Here's how the part is built. I have some questions about the finished solid (model axes, mm). A direction names the side the tool comes from. Give positions to 0.01 mm unless a question says otherwise; leave off trailing zeros. Loops run counter-clockwise (first coordinate to the right, second up) from the corner with the lowest first, then second, coordinate; pieces in that order, holes last. Notation, with made-up numbers: (5, 46.25) - (35, 46.25) arc R19 cw to (35, 65.25) - close; hole circle Ø4 at (50, 72.5). An arc over 180 degrees is marked (long way). Use a Markdown table: item, result.
from build123d import *

# Parameters (mm, degrees)
SKETCH2_W             = 40.64
SKETCH2_H             = 26.67
BOSS_EXTRUDE1_DEPTH   = 37.338
SKETCH3_R             = 3.7592
BODY_TUBE_CUT_DEPTH   = 62.294573528
SKETCH4_W             = 22.86
SKETCH4_H             = 18.288
SERVO_BODY_HOLE_DEPTH = 26.67
CUT_EXTRUDE3_REACH    = 63.295
SKETCH5_W             = 7.874
SKETCH5_H             = 9.144


with BuildPart() as part:
    # Sketch2 → Boss-Extrude1 (new body)
    with BuildSketch(Plane(origin=(0, 0, 0), x_dir=(1, 0, 0), z_dir=(0, 1, 0))):
        with Locations((20.32, 13.335)):
            Rectangle(SKETCH2_W, SKETCH2_H)
    extrude(amount=BOSS_EXTRUDE1_DEPTH)

    # Sketch3 → Body Tube Cut (cut, through all)
    with BuildSketch(Plane(origin=(40.64, 0, 0), x_dir=(0, 0, -1), z_dir=(1, 0, 0))):
        with Locations((13.335, 0)):
            Circle(SKETCH3_R)
    extrude(amount=-BODY_TUBE_CUT_DEPTH, mode=Mode.SUBTRACT)

    # Sketch4 → Servo Body Hole (cut)
    with BuildSketch(Plane.XY):
        with Locations((20.193, 19.558)):
            Rectangle(SKETCH4_W, SKETCH4_H)
    extrude(amount=-SERVO_BODY_HOLE_DEPTH, mode=Mode.SUBTRACT)

    # Cut-Extrude3: up to this face of the body (flat: up to its plane)
    cut_extrude3_end = Plane(part.part.faces().sort_by_distance((0, 19.058270015, -13.335))[0])
    # Sketch5 → Cut-Extrude3 (cut, up to the picked face)
    with BuildSketch(Plane(origin=(40.64, 0, 0), x_dir=(0, 0, -1), z_dir=(1, 0, 0)), mode=Mode.PRIVATE) as cut_extrude3_sk1:
        with Locations((3.937, 24.13)):
            Rectangle(SKETCH5_W, SKETCH5_H)
    cut_extrude3_tool1 = split(extrude(cut_extrude3_sk1.sketch, amount=-CUT_EXTRUDE3_REACH, mode=Mode.PRIVATE), bisect_by=cut_extrude3_end, keep=Keep.BOTH, mode=Mode.PRIVATE)
    # Sketch5 → Cut-Extrude3 (cut, up to the picked face)
    with BuildSketch(Plane(origin=(40.64, 0, 0), x_dir=(0, 0, -1), z_dir=(1, 0, 0)), mode=Mode.PRIVATE) as cut_extrude3_sk2:
        with Locations((22.733, 14.986)):
            Rectangle(SKETCH5_W, SKETCH5_H)
    cut_extrude3_tool2 = split(extrude(cut_extrude3_sk2.sketch, amount=-CUT_EXTRUDE3_REACH, mode=Mode.PRIVATE), bisect_by=cut_extrude3_end, keep=Keep.BOTH, mode=Mode.PRIVATE)
    add(cut_extrude3_tool1.solids().sort_by(Axis((40.64, 24.13, -3.937), (-1, 0, 0)))[0], mode=Mode.SUBTRACT)
    add(cut_extrude3_tool2.solids().sort_by(Axis((40.64, 14.986, -22.733), (-1, 0, 0)))[0], mode=Mode.SUBTRACT)


solid = part.part
(1) Suppose I cut it at D-D on x = 36.5. Write out the boundary of the cut face in (y, z) (3 decimals), plus the area to 3 significant figures.
A:
| item | result |
|---|---|
| outline | (0, -26.67) - (10.414, -26.67) - (10.414, -18.796) - (19.558, -18.796) - (19.558, -26.67) - (37.338, -26.67) - (37.338, 0) - (28.702, 0) - (28.702, -7.874) - (19.558, -7.874) - (19.558, 0) - (0, 0) - (0, -9.576) arc R3.759 cw to (0, -17.094) - close |
| area | 830 mm2 |
(2) Suppose I cut it at A-A on x = 25. Write out the boundary of the cut face in (y, z) (3 decimals), plus the area to 3 significant figures.
A:
| item | result |
|---|---|
| outline | (0, -26.67) - (10.414, -26.67) - (10.414, 0) - (0, 0) - (0, -9.576) arc R3.759 cw to (0, -17.094) - close; (28.702, -26.67) - (37.338, -26.67) - (37.338, 0) - (28.702, 0) - close |
| area | 486 mm2 |
(3) On a 3-axis mill with a long thin cutter (end or side, diameter ignored), from which of +Z, -Z, +X, -X, +Y, -Y can I reach the whole of each face in a straight line? I mean faces 1 (the face through (8.763, 19, -13)), 2 (the face through (4, 19.558, -23)), 3 (the face through (36, 19.558, -4)). Say none if no direction works.
A:
| item | result |
|---|---|
| face 1 | +Z, -Z |
| face 2 | -Z, +X, -X |
| face 3 | +Z, +X, -X |
(4) We'd pull the mould along X, two halves only. Please class faces 4 (the face through (36, 24, -7.874)), 5 (the face through (21, 28.702, -10)), 6 (the face through (40.64, 18, -13)): pulls with the +X half, pulls with the -X half, needs draft (parallel to the pull), parting line crosses it, or undercut.
A:
| item | result |
|---|---|
| face 4 | needs draft |
| face 5 | undercut |
| face 6 | pulls with the +X half |
(5) Will these pins go through, and if not, where does the flat tip stop? pin 1 (2 mm diameter, centred on x = 14.5, z = -19.5, fed in from -Y); pin 2 (2.5 mm diameter, centred on x = 35, y = 22, fed in from +Z); pin 3 (2.5 mm diameter, centred on x = 34.5, y = 13, fed in from -Z).
A:
| item | result |
|---|---|
| pin 1 | y = 0 |
| pin 2 | z = -7.87 |
| pin 3 | z = -18.8 |
(6) Suppose I cut it at C-C on y = 22. Write out the boundary of the cut face in (x, z).
A:
| item | result |
|---|---|
| outline | (0, -26.67) - (8.76, -26.67) - (8.76, -7.87) - (0, -7.87) - close; (31.62, -26.67) - (40.64, -26.67) - (40.64, -7.87) - (31.62, -7.87) - close |
(7) Suppose I cut it at B-B on z = -24.25. Write out the boundary of the cut face in (x, y).
A:
| item | result |
|---|---|
| outline | (0, 0) - (40.64, 0) - (40.64, 10.41) - (0, 10.41) - close; (0, 19.56) - (8.76, 19.56) - (8.76, 28.7) - (31.62, 28.7) - (31.62, 19.56) - (40.64, 19.56) - (40.64, 37.34) - (0, 37.34) - close |
(8) If I drill on line 1 (X direction, y = 16.5, z = -16); line 2 (Y direction, x = 21, z = -23); line 3 (Y direction, x = 36, z = -21), over which ranges is the centre line in solid material (lowest first)?
A:
| item | result |
|---|---|
| line 1 | 0 to 8.76, 31.62 to 40.64 |
| line 2 | 0 to 10.41, 28.7 to 37.34 |
| line 3 | 0 to 10.41, 19.56 to 37.34 |
